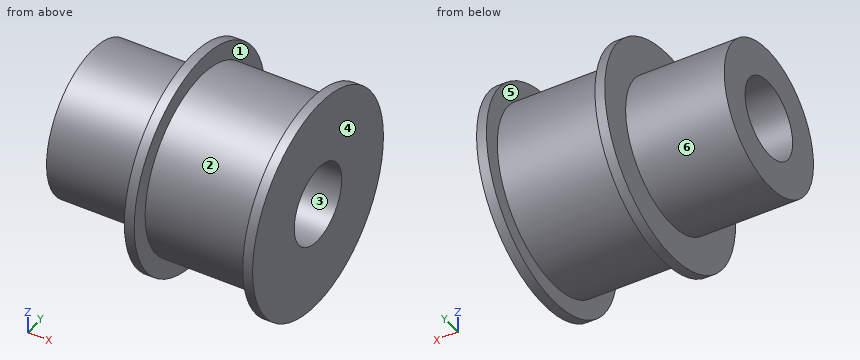
from build123d import *

# Parameters (mm, degrees)
SKETCH_1_R          = 11
EXTRUDE_1_DEPTH     = 13
SKETCH_2_R          = 11
SKETCH_2_R_2        = 9.17
CUT_EXTRUDE_1_DEPTH = 5.5
SKETCH_3_R          = 7.5
EXTRUDE_2_DEPTH     = 10
CUT_EXTRUDE_2_REACH = 29.767
SKETCH_4_R          = 4


with BuildPart() as part:
    # 草图1 → 凸台-拉伸1 (new body)
    with BuildSketch(Plane(origin=(0, 0, 0), x_dir=(0, 0, -1), z_dir=(1, 0, 0))):
        with Locations(Location((0, 0, 0), (0, 0, 180))):
            Circle(SKETCH_1_R)
    extrude(amount=EXTRUDE_1_DEPTH)

    # 草图2 → 切除-拉伸1 (cut, symmetric)
    with BuildSketch(Plane(origin=(6.5, 0, 0), x_dir=(0, 0, -1), z_dir=(1, 0, 0))):
        with Locations(Location((0, 0, 0), (0, 0, 180))):
            Circle(SKETCH_2_R)
        Circle(SKETCH_2_R_2, mode=Mode.SUBTRACT)
    extrude(amount=CUT_EXTRUDE_1_DEPTH, both=True, mode=Mode.SUBTRACT)

    # 草图3 → 凸台-拉伸2 (add)
    with BuildSketch(Plane.ZY):
        Circle(SKETCH_3_R)
    extrude(amount=EXTRUDE_2_DEPTH)

    # 草图4 → 切除-拉伸2 (cut, up to next)
    with BuildSketch(Plane.ZY.offset(10), mode=Mode.PRIVATE) as cut_extrude_2_sk1:
        Circle(SKETCH_4_R)
    cut_extrude_2_tool1 = extrude(cut_extrude_2_sk1.sketch, amount=-CUT_EXTRUDE_2_REACH, mode=Mode.PRIVATE) & part.part
    add(cut_extrude_2_tool1.solids().sort_by_distance((-10, 0, 0))[0], mode=Mode.SUBTRACT)


solid = part.part
Here's how the part is built. I have some questions about the finished solid (model axes, mm). Face numbers are marked on the shaded views. A direction names the side the tool comes from. Coordinates: 2 decimals unless noted, no trailing zeros. Write each loop counter-clockwise with the first axis right and the second up, starting at its lowest first coordinate (ties: lowest second). Pieces come first, ordered by that corner, then holes.
1) If we section it at A-A (y = 0): List the corners of the cut face in (x, z) for me.
Filled in:
outline: (-10, -7.5) - (0, -7.5) - (0, -11) - (1, -11) - (1, -9.17) - (12, -9.17) - (12, -11) - (13, -11) - (13, -4) - (-10, -4) - close; (-10, 4) - (13, 4) - (13, 11) - (12, 11) - (12, 9.17) - (1, 9.17) - (1, 11) - (0, 11) - (0, 7.5) - (-10, 7.5) - close
2) If we section it at C-C (x = -5): List the corners of the cut face in (y, z) for me, plus the area to 3 significant figures.
Filled in:
outline: circle Ø15 at (0, 0); hole circle Ø8 at (0, 0)
area: 126 mm2
3) Which directions (+Z, -Z, +X, -X, +Y, -Y) give clear straight access to the entire face, cutting with the end or side of a thin tool? Please do the marked faces 4, 5 and 6.
Filled in:
face 4: +Z, -Z, +X, +Y, -Y
face 5: none
face 6: -X
4) If I drill on line 1 (Y direction, x = -1.5, z = 0); line 2 (X direction, y = -8.25, z = 4.75); line 3 (X direction, y = 6.75, z = 5.75), over which ranges is the centre line in solid material (lowest first)?
Filled in:
line 1: y = -7.5 to -4, 4 to 7.5
line 2: x = 0 to 1, 12 to 13
line 3: x = 0 to 13
5) I'm going to push flat-ended pins straight in: pin 1 (6 mm diameter, centred on x = 3.5, z = 8.5, fed in from -Y); pin 2 (3 mm diameter, centred on x = 1, y = 3, fed in from -Z); pin 3 (8 mm diameter, centred on x = 3.5, z = 5.5, fed in from +Y). Where does each tip first touch, or does it pass through?
Filled in:
pin 1: stops at y = -8.61
pin 2: stops at z = -10.9
pin 3: stops at y = 10.74
6) Thinking about a two-plate mould opening in Y: for the marked faces 1, 2 and 3, which applies, +Y half, -Y half, draft (parallel to the pull), parting line (faces both ways), or undercut?
Filled in:
face 1: draft
face 2: parting line
face 3: undercut
7) If we section it at D-D (z = 7): List the corners of the cut face in (x, y) for me.
Filled in:
outline: (-10, -2.69) - (0, -2.69) - (0, -8.49) - (1, -8.49) - (1, -5.92) - (12, -5.92) - (12, -8.49) - (13, -8.49) - (13, 8.49) - (12, 8.49) - (12, 5.92) - (1, 5.92) - (1, 8.49) - (0, 8.49) - (0, 2.69) - (-10, 2.69) - close
